Check sheet for the modelled part. Datum: model origin and axes. Units: mm. Give positions to 0.01 mm unless a question says otherwise; leave off trailing zeros. Write each loop counter-clockwise with the first axis right and the second up, starting at its lowest first coordinate (ties: lowest second). Pieces come first, ordered by that corner, then holes. Notation, with made-up numbers: (-1.5, 42) -> (42.5, 42) arc R23 ccw to (42.5, 76) -> close; hole circle Ø8 at (88, 20). An arc over 180 degrees is marked (long way). Use a Markdown table: item, result. Add a question column.
1. Cross-section at A-A (x = 3). Enter the section's corners in (y, z), then the cut area to 3 significant figures.
2. Scan lines: probe 1 along X at (y, z) = (1.65, -1); probe 2 along Z at (x, y) = (14, 0.75). Record each from-to range of solid material in increasing order. Write a range as [from, to].
3. Cross-section at B-B (y = 0.8). Enter the section's corners in (x, z).
4. Cross-section at C-C (z = -5.5). Enter the section's corners in (x, y).
Autodesk Inventor part; units mm, degrees
ref_plane "YZ Plane" through (0, 0, 0) normal (1, 0, 0) x (0, 1, 0)
ref_plane "XZ Plane" through (0, 0, 0) normal (0, 1, 0) x (-1, 0, 0)
ref_plane "XY Plane" through (0, 0, 0) normal (0, 0, 1) x (1, 0, 0)
sketch "스케치1" plane through (0, 0, 0) normal (0, 1, 0) x (-1, 0, 0)
  line L0 (-32.5919, 13.5) -> (-13.5, 32.5919)
  line L1 (-13.5, 32.5919) -> (13.5, 32.5919)
  line L2 (13.5, 32.5919) -> (32.5919, 13.5)
  line L3 (32.5919, 13.5) -> (32.5919, -13.5)
  line L4 (32.5919, -13.5) -> (13.5, -32.5919)
  line L5 (13.5, -32.5919) -> (-13.5, -32.5919)
  line L6 (-13.5, -32.5919) -> (-32.5919, -13.5)
  line L7 (-32.5919, -13.5) -> (-32.5919, 13.5)
  line L8 (21.0459, 13.5) -> (21.0459, -13.5)
  line L9 (-21.0459, -13.5) -> (-21.0459, 13.5)
  line L10 (13.5, -21.0459) -> (-13.5, -21.0459)
  line L11 (-13.5, 21.0459) -> (13.5, 21.0459)
  line L12 (13.5, -21.0459) -> (21.0459, -13.5)
  line L13 (21.0459, 13.5) -> (13.5, 21.0459)
  line L14 (-13.5, 21.0459) -> (-21.0459, 13.5)
  line L15 (-21.0459, -13.5) -> (-13.5, -21.0459)
  point P0 (0, 0)
  point P1 (0, 0)
  point P2 (0, 21.0459)
  point P3 (0, -32.5919)
  dimension "d0" = 27
  dimension "d1" = 11.546
  dimension "d2" = 11.546
  dimension "d3" = 11.546
  dimension "d4" = 11.546
extrude "돌출1" add sketch "스케치1" along normal blind 2 contours L8 L12 L10 L15 L9 L14 L11 L13
shell "쉘1" thickness 0.8 removed faces 2 at (7.0153, 0, 4.5) at (7.0153, 2, 4.5)
properties part number "팔각형 OV-PAM 5패턴 층 한개 부피 구하기 0도 - 수정"
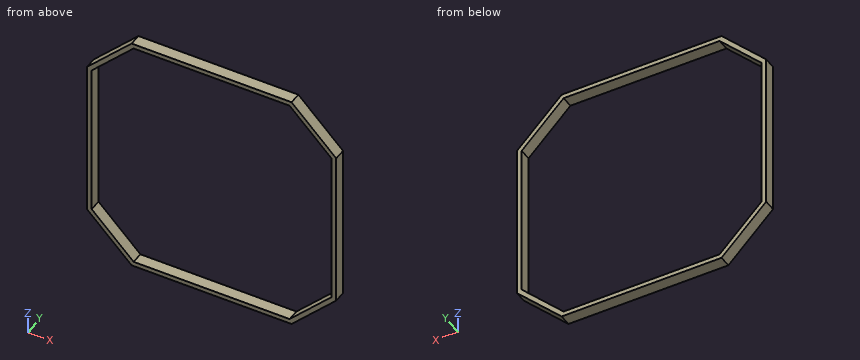
Worked answers:
| question | item | result |
|---|---|---|
| 1 | outline | (0, -21.05) -> (2, -21.05) -> (2, -20.25) -> (0, -20.25) -> close; (0, 20.25) -> (2, 20.25) -> (2, 21.05) -> (0, 21.05) -> close |
| 1 | area | 3.20 mm² |
| 2 | probe 1 | x = [-21.05, -20.25], [20.25, 21.05] |
| 2 | probe 2 | z = [-20.55, -19.41], [19.41, 20.55] |
| 3 | outline | (-21.05, -13.5) -> (-13.5, -21.05) -> (13.5, -21.05) -> (21.05, -13.5) -> (21.05, 13.5) -> (13.5, 21.05) -> (-13.5, 21.05) -> (-21.05, 13.5) -> close; hole (-20.25, -13.17) -> (-13.17, -20.25) -> (13.17, -20.25) -> (20.25, -13.17) -> (20.25, 13.17) -> (13.17, 20.25) -> (-13.17, 20.25) -> (-20.25, 13.17) -> close |
| 4 | outline | (-21.05, 0) -> (-20.25, 0) -> (-20.25, 2) -> (-21.05, 2) -> close; (20.25, 0) -> (21.05, 0) -> (21.05, 2) -> (20.25, 2) -> close |
